from build123d import *

# Parameters (mm, degrees)
SKETCH1_W           = 50.8
SKETCH1_H           = 12.7
BOSS_EXTRUDE1_DEPTH = 6.35
BOSS_EXTRUDE2_DEPTH = 12.7


with BuildPart() as part:
    # Sketch1 → Boss-Extrude1 (new body)
    with BuildSketch(Plane.XY):
        with Locations((25.4, 6.35)):
            Rectangle(SKETCH1_W, SKETCH1_H)
    extrude(amount=BOSS_EXTRUDE1_DEPTH)

    # Sketch4 → Boss-Extrude2 (add)
    with BuildSketch(Plane.XZ):
        with BuildLine():
            Line((18.953484491, 6.35), (31.653484491, 6.35))
            Line((31.653484491, 6.35), (31.653484491, 57.15))
            ThreePointArc((31.653484491, 57.15), (25.303484491, 63.5), (18.953484491, 57.15))
            Line((18.953484491, 57.15), (18.953484491, 6.35))
        make_face()
        with BuildLine():
            Line((22.117326524, 57.65327603), (22.117326524, 19.05))
            Line((22.117326524, 19.05), (28.605484491, 19.05))
            Line((28.605484491, 19.05), (28.605484491, 57.65327603))
            ThreePointArc((28.605484491, 57.65327603), (25.361405508, 60.897355013), (22.117326524, 57.65327603))
        make_face(mode=Mode.SUBTRACT)
    extrude(amount=-BOSS_EXTRUDE2_DEPTH)


solid = part.part
For this review, take the finished solid that the model builds, in its own axes (mm). A direction names the side the tool comes from. Round coordinates to 2 decimals unless told otherwise and drop trailing zeros. Loops run counter-clockwise (first coordinate to the right, second up) from the corner with the lowest first, then second, coordinate; pieces in that order, holes last. Notation, with made-up numbers: (24.25, -33.75) - (81.25, -33.75) arc R12 ccw to (81.25, -17.75) - close; hole circle Ø9 at (3, 89). An arc over 180 degrees is marked (long way). Use one line per item in the form item = value.
1) Tool access review of faces 5 (the face through (18.953, 6, 32)), 6 (the face through (25, 6, 0)), 7 (the face through (31.653, 6, 31)), 8 (the face through (25, 6, 19.05)), 9 (the face through (50.8, 6, 3)): name each direction out of +Z, -Z, +X, -X, +Y, -Y from which nothing blocks a thin tool from reaching the whole face with its end or side.
Solutions:
face_5 = +Z, -X, +Y, -Y
face_6 = -Z, +X, -X, +Y, -Y
face_7 = +Z, +X, +Y, -Y
face_8 = +Y, -Y
face_9 = +Z, -Z, +X, +Y, -Y
2) We need section D-D on z = 10. Write out the cut boundary in (x, y).
Solutions:
outline = (18.95, 0) - (31.65, 0) - (31.65, 12.7) - (18.95, 12.7) - close
3) We need section A-A on z = 51. Write out the cut boundary in (x, y), then the cut area to 3 significant figures.
Solutions:
outline = (18.95, 0) - (22.12, 0) - (22.12, 12.7) - (18.95, 12.7) - close; (28.61, 0) - (31.65, 0) - (31.65, 12.7) - (28.61, 12.7) - close
area = 78.9 mm2
4) Wall thickness on probe 1 along X at (y, z) = (9, 29.5); probe 2 along Z at (x, y) = (14.5, 3); probe 3 along X at (y, z) = (1, 16): over which ranges is each line inside the solid? List them lowest first.
Solutions:
probe_1 = 18.95 to 22.12, 28.61 to 31.65
probe_2 = 0 to 6.35
probe_3 = 18.95 to 31.65
5) Mouldability with a two-part tool opening along X and no side actions: class faces 1 (the face through (22.117, 6, 39)), 2 (the face through (41, 6, 6.35)), 3 (the face through (0, 6, 3)), 4 (the face through (25.433, 6.261, 60.897)) as pulls with the +X half, pulls with the -X half, needs draft (parallel to the pull), parting line crosses it, or undercut.
Solutions:
face_1 = undercut
face_2 = needs draft
face_3 = pulls with the -X half
face_4 = undercut
6) We need section C-C on x = 39.5. Write out the cut boundary in (y, z), then the cut area to 3 significant figures.
Solutions:
outline = (0, 0) - (12.7, 0) - (12.7, 6.35) - (0, 6.35) - close
area = 80.6 mm2
7) Clearance check with flat-ended pins moving along their axes: P1, Ø6.5, axis at x = 39, y = 5, coming from the +Z side; P2, Ø6.5, axis at y = 7.5, z = 47.5, coming from the +X side. State where each tip first meets the part, or that it passes through.
Solutions:
P1 = 6.35
P2 = 31.65
8) We need section B-B on y = 5.5. Write out the cut boundary in (x, z).
Solutions:
outline = (0, 0) - (50.8, 0) - (50.8, 6.35) - (31.65, 6.35) - (31.65, 57.15) arc R6.35 ccw to (18.95, 57.15) - (18.95, 6.35) - (0, 6.35) - close; hole (22.12, 19.05) - (28.61, 19.05) - (28.61, 57.65) arc R3.24 ccw to (22.12, 57.65) - close
